from build123d import *

# Parameters (mm, degrees)
SKETCH1_R           = 1.9
SKETCH1_R_2         = 1
BOSS_EXTRUDE1_DEPTH = 7
SKETCH2_R           = 1.9
SKETCH2_R_2         = 1.4
CUT_EXTRUDE1_DEPTH  = 3.5
SKETCH3_R           = 1
BOSS_EXTRUDE2_DEPTH = 3.5


with BuildPart() as part:
    # Sketch1 → Boss-Extrude1 (new body)
    with BuildSketch(Plane.XY):
        Circle(SKETCH1_R)
        Circle(SKETCH1_R_2, mode=Mode.SUBTRACT)
    extrude(amount=-BOSS_EXTRUDE1_DEPTH)

    # Sketch2 → Cut-Extrude1 (cut)
    with BuildSketch(Plane.XY):
        Circle(SKETCH2_R)
        Circle(SKETCH2_R_2, mode=Mode.SUBTRACT)
    extrude(amount=-CUT_EXTRUDE1_DEPTH, mode=Mode.SUBTRACT)

    # Sketch3 → Boss-Extrude2 (add)
    with BuildSketch(Plane.XY):
        with BuildLine():
            Line((1.579792263, 1.055583443), (1.767766953, 1.767766953))
            Line((1.767766953, 1.767766953), (1.055583443, 1.579792263))
            Line((1.055583443, 1.579792263), (0.659955432, 1.23468977))
            ThreePointArc((0.659955432, 1.23468977), (0.598577131, 1.26558501), (0.535756805, 1.293431346))
            ThreePointArc((0.535756805, 1.293431346), (0.471645795, 1.318161691), (0.406398548, 1.33971647))
            Line((0.406398548, 1.33971647), (0.370671612, 1.863492033))
            Line((0.370671612, 1.863492033), (0, 2.5))
            Line((0, 2.5), (-0.370671612, 1.863492033))
            Line((-0.370671612, 1.863492033), (-0.406398548, 1.33971647))
            ThreePointArc((-0.406398548, 1.33971647), (-0.471645795, 1.318161691), (-0.535756805, 1.293431346))
            ThreePointArc((-0.535756805, 1.293431346), (-0.598577131, 1.26558501), (-0.659955432, 1.23468977))
            Line((-0.659955432, 1.23468977), (-1.055583443, 1.579792263))
            Line((-1.055583443, 1.579792263), (-1.767766953, 1.767766953))
            Line((-1.767766953, 1.767766953), (-1.579792263, 1.055583443))
            Line((-1.579792263, 1.055583443), (-1.23468977, 0.659955432))
            ThreePointArc((-1.23468977, 0.659955432), (-1.26558501, 0.598577131), (-1.293431346, 0.535756805))
            ThreePointArc((-1.293431346, 0.535756805), (-1.318161691, 0.471645795), (-1.33971647, 0.406398548))
            Line((-1.33971647, 0.406398548), (-1.863492033, 0.370671612))
            Line((-1.863492033, 0.370671612), (-2.5, 0))
            Line((-2.5, 0), (-1.863492033, -0.370671612))
            Line((-1.863492033, -0.370671612), (-1.33971647, -0.406398548))
            ThreePointArc((-1.33971647, -0.406398548), (-1.318161691, -0.471645795), (-1.293431346, -0.535756805))
            ThreePointArc((-1.293431346, -0.535756805), (-1.26558501, -0.598577131), (-1.23468977, -0.659955432))
            Line((-1.23468977, -0.659955432), (-1.579792263, -1.055583443))
            Line((-1.579792263, -1.055583443), (-1.767766953, -1.767766953))
            Line((-1.767766953, -1.767766953), (-1.055583443, -1.579792263))
            Line((-1.055583443, -1.579792263), (-0.659955432, -1.23468977))
            ThreePointArc((-0.659955432, -1.23468977), (-0.598577131, -1.26558501), (-0.535756805, -1.293431346))
            ThreePointArc((-0.535756805, -1.293431346), (-0.471645795, -1.318161691), (-0.406398548, -1.33971647))
            Line((-0.406398548, -1.33971647), (-0.370671612, -1.863492033))
            Line((-0.370671612, -1.863492033), (0, -2.5))
            Line((0, -2.5), (0.370671612, -1.863492033))
            Line((0.370671612, -1.863492033), (0.406398548, -1.33971647))
            ThreePointArc((0.406398548, -1.33971647), (0.471645795, -1.318161691), (0.535756805, -1.293431346))
            ThreePointArc((0.535756805, -1.293431346), (0.598577131, -1.26558501), (0.659955432, -1.23468977))
            Line((0.659955432, -1.23468977), (1.055583443, -1.579792263))
            Line((1.055583443, -1.579792263), (1.767766953, -1.767766953))
            Line((1.767766953, -1.767766953), (1.579792263, -1.055583443))
            Line((1.579792263, -1.055583443), (1.23468977, -0.659955432))
            ThreePointArc((1.23468977, -0.659955432), (1.26558501, -0.598577131), (1.293431346, -0.535756805))
            ThreePointArc((1.293431346, -0.535756805), (1.318161691, -0.471645795), (1.33971647, -0.406398548))
            Line((1.33971647, -0.406398548), (1.863492033, -0.370671612))
            Line((1.863492033, -0.370671612), (2.5, 0))
            Line((2.5, 0), (1.863492033, 0.370671612))
            Line((1.863492033, 0.370671612), (1.33971647, 0.406398548))
            ThreePointArc((1.33971647, 0.406398548), (1.318161691, 0.471645795), (1.293431346, 0.535756805))
            ThreePointArc((1.293431346, 0.535756805), (1.26558501, 0.598577131), (1.23468977, 0.659955432))
            Line((1.23468977, 0.659955432), (1.579792263, 1.055583443))
        make_face()
        Circle(SKETCH3_R, mode=Mode.SUBTRACT)
    extrude(amount=-BOSS_EXTRUDE2_DEPTH)


solid = part.part
The model under review builds one solid part; all positions refer to its coordinate system, in mm. Round coordinates to 2 decimals unless told otherwise and drop trailing zeros. Loops run counter-clockwise (first coordinate to the right, second up) from the corner with the lowest first, then second, coordinate; pieces in that order, holes last. Notation, with made-up numbers: M 15.25,-7 L 20.25,-7 A27 cw 20.25,29 Z; hole C 69.5,33.25 d3. An arc over 180 degrees is marked long. Answer as CSV lines item,"result". Start each with the question number.
Item 1: Wall thickness on line 1 (Y direction, x = 0, z = -5); line 2 (Z direction, x = 1.75, y = 0.5); line 3 (Z direction, x = 1.7, y = -1.65): over which ranges is each line inside the solid? List them lowest first. Write a range as [from, to].
Item 2: Mouldability with a two-part tool opening along X and no side actions: class faces 1 (the face through (-1.9, 0.08, -5.23)), 2 (the face through (0, -1, -3)), 3 (the face through (1, -1, -7)) as released by +X, released by -X, zero draft, split by the parting line, or undercut.
Item 3: Consider section A-A (z = -5.25). Write out the cut boundary in (x, y).
Item 4: Insertion check: P1, Ø1.5, axis at x = 0, z = -2.5, coming from the -Y side; P2, Ø2, axis at y = -1.5, z = -5, coming from the +X side. Each pin has a flat end and moves straight along its axis. Give the tip position at first contact, or say it passes through.
Answer:
1,line 1,"y = [-1.9, -1], [1, 1.9]"
1,line 2,"z = [-7, -3.5]"
1,line 3,"z = [-3.5, 0]"
2,face 1,"split by the parting line"
2,face 2,"undercut"
2,face 3,"zero draft"
3,outline,"C 0,0 d3.8; hole C 0,0 d2"
4,P1,"stops at y = -2.5"
4,P2,"stops at x = 1.83"
